Geometry check sheet. Reference: the model listing, model coordinates, mm. Face numbers are marked on the shaded views. Coordinates: 2 decimals unless noted, no trailing zeros. Loops run counter-clockwise (first coordinate to the right, second up) from the corner with the lowest first, then second, coordinate; pieces in that order, holes last. Notation, with made-up numbers: (-4.75, 60) -> (19.25, 60) arc R18 ccw to (19.25, 67) -> close; hole circle Ø8 at (8, 58). An arc over 180 degrees is marked (long way). Answer as a JSON object with one key per item and string values.
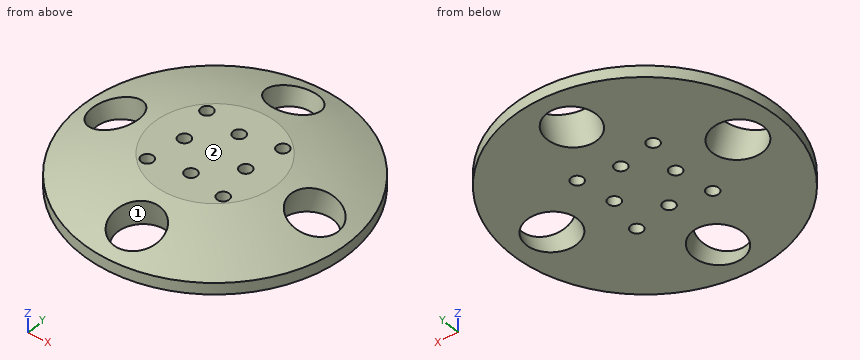
from build123d import *

# Parameters (mm, degrees)
PATTERN_CIRCULAR_1_COUNT = 4
SKETCH_3_R               = 1.6
CUT_EXTRUDE_1_DEPTH      = 10
MOVE_BODY_4_ANGLE        = 90


with BuildPart() as part:
    # 草图1 → 旋转1 (revolve)
    with BuildSketch(Plane(origin=(0, 0, 0), x_dir=(0, 0, -1), z_dir=(1, 0, 0)), mode=Mode.PRIVATE) as revolve_1_sk:
        with BuildLine():
            Line((35.2879411, -15.710089558), (0, -15.710089558))
            Line((0, -15.710089558), (0, -7.210089558))
            Line((0, -7.210089558), (16.237996189, -7.210089558))
            ThreePointArc((16.237996189, -7.210089558), (25.906639592, -9.432422882), (35.2879411, -12.6592809))
            Line((35.2879411, -12.6592809), (35.2879411, -15.710089558))
        make_face()
    revolve(revolve_1_sk.sketch.rotate(Axis((0, 31.276946121, 0), (0, -1, 0)), 180), axis=Axis((0, 31.276946121, 0), (0, -1, 0)))

    # 草图2 → 切除-旋转1 (revolve, cut)
    with BuildSketch(Plane(origin=(0, 0, 0), x_dir=(0, 0, -1), z_dir=(1, 0, 0)), mode=Mode.PRIVATE) as cut_revolve_1_sk:
        Polygon((30.059364586, 4.546712214), (36.307565609, 2.755069401), (21.502083986, -48.87778106), (15.253882963, -47.086138247), align=None)
    cut_revolve_1 = revolve(cut_revolve_1_sk.sketch.rotate(Axis((0, -100.021482202, -0.07491734), (0, 0.9612616959383208, -0.27563735581699245)), 33.246351954), axis=Axis((0, -100.021482202, -0.07491734), (0, 0.9612616959383208, -0.27563735581699245)), mode=Mode.SUBTRACT)

    # 阵列(圆周)1: 切除-旋转1 ×4 about axis
    pattern_circular_1_axis = Axis((0, -7.210089558, 0), (0, 1, 0))
    for i in range(1, PATTERN_CIRCULAR_1_COUNT):
        add(cut_revolve_1.rotate(pattern_circular_1_axis, i * 360 / PATTERN_CIRCULAR_1_COUNT), mode=Mode.SUBTRACT)

    # 草图3 → 切除-拉伸1 (cut)
    with BuildSketch(Plane.XZ.offset(15.710089558)):
        with Locations(Location((8, 0, 0), (0, 0, 270))):
            Circle(SKETCH_3_R)
        with Locations(Location((0, 8, 0), (0, 0, 270))):
            Circle(SKETCH_3_R)
        with Locations(Location((0, -8, 0), (0, 0, 270))):
            Circle(SKETCH_3_R)
        with Locations(Location((-8, 0, 0), (0, 0, 270))):
            Circle(SKETCH_3_R)
        with Locations(Location((9.899494937, -9.899494937, 0), (0, 0, 270))):
            Circle(SKETCH_3_R)
        with Locations(Location((-9.899494937, -9.899494937, 0), (0, 0, 270))):
            Circle(SKETCH_3_R)
        with Locations(Location((-9.899494937, 9.899494937, 0), (0, 0, 270))):
            Circle(SKETCH_3_R)
        with Locations(Location((9.899494937, 9.899494937, 0), (0, 0, 270))):
            Circle(SKETCH_3_R)
    extrude(amount=-CUT_EXTRUDE_1_DEPTH, mode=Mode.SUBTRACT)


with BuildPart() as part_1:
    # Move Body 4: moved
    add(part.part.rotate(Axis((0, -11.460089558, 0), (1, 0, 0)), MOVE_BODY_4_ANGLE))


solid = part_1.part
1. Section check C-C, the plane z = 2.25. State how many separate pieces and enclosed holes the cut face has, then the cut area to 3 significant figures.
Evaluation:
{"separate pieces": "1", "enclosed holes": "8", "area": "1,710 mm^2"}
2. Mould release check, pull along X, two halves, no side actions. Record for the marked faces 1 and 2: released by +X, released by -X, zero draft, split by the parting line, or undercut.
Evaluation:
{"face 1": "undercut", "face 2": "zero draft"}
3. Thickness scan on probe 1 along Y at (x, z) = (1, -2); probe 2 along X at (y, z) = (-17, -1.25); probe 3 along Y at (x, z) = (-4, -3). Record the ranges inside material, lowest first. Write a range as from..to.
Evaluation:
{"probe 1": "y = -46.73..-43.04, -29.67..-20.71, -18.21..-4.71, -2.21..6.75, 20.12..23.81", "probe 2": "x = -34.85..-28.65, -21.57..21.57, 28.65..34.85", "probe 3": "y = -46.52..-41.4, -30.74..7.82, 18.48..23.6"}
4. Section check A-A, the plane y = -7. Record the boundary of the cut face in (x, z), then the cut area to 3 significant figures.
Evaluation:
{"outline": "(-35, -4.25) -> (-29.17, -4.25) -> (-30.52, 0.47) arc R94.09 ccw to (-35, -1.2) -> close; (-21.43, 3.08) -> (-19.33, -4.25) -> (19.33, -4.25) -> (21.43, 3.08) arc R94.09 ccw to (15.61, 4.25) -> (-15.61, 4.25) arc R94.09 ccw to start; (29.17, -4.25) -> (35, -4.25) -> (35, -1.2) arc R94.09 ccw to (30.52, 0.47) -> close", "area": "384 mm^2"}
5. Depth check by flat-ended pin: P1, Ø5, axis at x = 27, z = -1.5, coming from the -Y side; P2, Ø3, axis at x = 8, y = -11.46, coming from the -Z side; P3, Ø1.5, axis at y = 6, z = -2.5, coming from the -X side. Enter the tip coordinate at first touch or a pass-through.
Evaluation:
{"P1": "stops at y = -36.86", "P2": "passes through", "P3": "stops at x = -31.08"}
6. Section check B-B, the plane x = 0. Record the boundary of the cut face in (y, z), then the cut area to 3 significant figures.
Evaluation:
{"outline": "(-46.75, -4.25) -> (-42.47, -4.25) -> (-43.68, -0.02) arc R94.2 ccw to (-46.75, -1.2) -> close; (-31.19, 3.57) -> (-28.95, -4.25) -> (-21.06, -4.25) -> (-21.06, 4.25) -> (-27.7, 4.25) arc R94.2 ccw to start; (-17.86, -4.25) -> (-5.06, -4.25) -> (-5.06, 4.25) -> (-17.86, 4.25) -> close; (-1.86, -4.25) -> (6.03, -4.25) -> (8.27, 3.57) arc R94.2 ccw to (4.78, 4.25) -> (-1.86, 4.25) -> close; (19.55, -4.25) -> (23.83, -4.25) -> (23.83, -1.2) arc R94.2 ccw to (20.76, -0.02) -> close", "area": "289 mm^2"}
